Build history of the part. All positions in model axes, mm. Give positions to 0.01 mm unless a question says otherwise; leave off trailing zeros. Order: outer loops, then holes, each group sorted by start corner. A loop starts at its lowest first (then second) coordinate and runs counter-clockwise, first axis right, second up. Notation, with made-up numbers: (34.25, -19) - (56.25, -19) arc R17 cw to (56.25, 4) - close; hole circle Ø8 at (26, -17.75). An arc over 180 degrees is marked (long way). One line per item, written item: value.
```python
from build123d import *

# Parameters (mm, degrees)
F0_W     = 185.6569993703
F0_H     = 254
F1_DEPTH = 254
F3_DEPTH = 254.001
F5_DEPTH = 80.8801199059
F6_DEPTH = 80.8801199059
F7_DEPTH = 132.7040067302


with BuildPart() as f1:
    # F0 (on Front) → F1 (new body)
    with BuildSketch(Plane.XZ):
        with Locations((92.8284996852, 127)):
            Rectangle(F0_W, F0_H)
    extrude(amount=F1_DEPTH)

    # F2 (on face) → F3 (cut, through all)
    with BuildSketch(Plane.XZ.offset(254)):
        Polygon((127, 0), (104.7778794644, 254), (0, 254), (0, 0), align=None)
    extrude(amount=-F3_DEPTH, mode=Mode.SUBTRACT)

    # F4 (on face) → F5 (cut, through all)
    with BuildSketch(Plane.YZ.offset(185.6569993703)):
        Polygon((-254, 254), (-254, 0), (-148.7897551572, 254), align=None)
    extrude(amount=-F5_DEPTH, mode=Mode.SUBTRACT)

    # F4 (on face) → F6 (cut, through all)
    with BuildSketch(Plane.YZ.offset(185.6569993703)):
        Polygon((-121.2969932698, 254), (-226.5072381126, 0), (0, 0), (0, 254), align=None)
    extrude(amount=-F6_DEPTH, mode=Mode.SUBTRACT)

    # F2 (on face) → F7 (cut, through all)
    with BuildSketch(Plane.XZ.offset(254)):
        Polygon((185.6569993703, 254), (130.274903338, 254), (152.4970238736, 0), (185.6569993703, 0), align=None)
    extrude(amount=-F7_DEPTH, mode=Mode.SUBTRACT)


solid = f1.part
```
(1) Slice it at B-B, the plane x = 145.5. Give the cut face in (y, z).
Completed:
outline: (-254, 0) - (-226.51, 0) - (-193.38, 79.98) - (-220.87, 79.98) - close
(2) Pin check, flat tips, straight feed: P1, Ø3, axis at y = -164.5, z = 207, coming from the +X side; P2, Ø3, axis at x = 120.5, z = 137, coming from the -Y side. Stop position of each tip, or through.
Completed:
P1: x = 134.52
P2: y = -197.87
(3) Drill centre lines: line 1 (Y direction, x = 124, z = 99.5); line 2 (Y direction, x = 125.5, z = 184.5); line 3 (X direction, y = -177, z = 162). Where is each one in solid material? Low to high.
Completed:
line 1: -212.79 to -185.29
line 2: -177.58 to -150.08
line 3: 112.83 to 138.32
(4) Slice it at A-A, the plane y = -230. Give the cut face in (x, z), and give its area (3 significant figures).
Completed:
outline: (121.93, 57.94) - (127, 0) - (152.5, 0) - (147.43, 57.94) - close
area: 1,480 mm²
